Work out the finished part from the listing and answer in its coordinate system (mm). A direction names the side the tool comes from. Round coordinates to 2 decimals unless told otherwise and drop trailing zeros. Order: outer loops, then holes, each group sorted by start corner. A loop starts at its lowest first (then second) coordinate and runs counter-clockwise, first axis right, second up. Notation, with made-up numbers: (82, 39) - (114, 39) arc R20 ccw to (114, 63) - close; hole circle Ø9 at (76, 82). An arc over 180 degrees is marked (long way). Put each result on its own line as item: value.
Solid Edge part; units mm, degrees
sketch "Sketch1" plane through (0, 0, 0) normal (1, 0, 0) x (0, 1, 0)
  circle A0 centre (0, 0) radius 30
  circle A1 centre (0, 0) radius 15
extrude "Protrusion1" add sketch "Sketch1" along normal mid plane 80
sketch "Sketch2" plane through (0, 0, 66) normal (0, 0, 1) x (1, 0, 0)
  line L0 (30, 0) -> (30, 40)
  line L1 (-30, 0) -> (-30, 40)
  line L2 (0, 0) -> (-30, 0)
  line L3 (0, 0) -> (30, 0)
  arc A0 (-30, 40) -> (30, 40) centre (0, 40) cw
extrude "ExtrudedProtrusion_3" add sketch "Sketch2" against normal blind 20
sketch "Sketch3" plane through (0, 0, 0) normal (1, 0, 0) x (0, 1, 0)
  line L0 (0, 46) -> (0, 0)
  line L1 (0, 0) -> (20.4926, 0)
  line L2 (20.4926, 0) -> (20, 22.3607)
  line L3 (20, 46) -> (20, 22.3607)
  line L4 (0, 46) -> (20, 46)
extrude "ExtrudedProtrusion_4" add sketch "Sketch3" along normal mid plane 60
sketch "Sketch4" plane through (0, 0, 0) normal (1, 0, 0) x (0, 1, 0)
  line L0 (0, 66) -> (-26.7217, 13.6364)
  line L1 (-26.7217, 13.6364) -> (-26.7217, 0)
  line L2 (-26.7217, 0) -> (0, 0)
  line L3 (0, 0) -> (0, 66)
extrude "ExtrudedProtrusion_5" add sketch "Sketch4" along normal mid plane 12
sketch "Sketch5" plane through (0, 0, 0) normal (1, 0, 0) x (0, 1, 0)
  circle A0 centre (0, 0) radius 15
extrude "ExtrudedCutout_2" cut sketch "Sketch5" along normal mid plane 321.4657
sketch "Sketch6" plane through (0, 0, 0) normal (1, 0, 0) x (0, 1, 0)
  line L0 (40, 106) -> (60, 106)
  line L1 (60, 106) -> (70, 66)
  line L2 (70, 66) -> (40, 66)
  line L3 (40, 66) -> (40, 106)
revolve "RevolvedProtrusion1" add sketch "Sketch6" angle 360 about axis through (0, 40, 66) along (0, 0, 1)
sketch "Sketch7" plane through (0, 0, 0) normal (1, 0, 0) x (0, 1, 0)
  line L0 (60, 66) -> (50, 106)
  line L1 (50, 106) -> (40, 106)
  line L2 (40, 106) -> (40, 66)
  line L3 (40, 66) -> (60, 66)
revolve "RevolvedCutout1" cut sketch "Sketch7" angle 360 about axis through (0, 40, 106) along (0, 0, -1)
1) A cutting plane is placed at C-C on y = 4. Write down the section's boundary in (x, z).
Findings below:
outline: (-40, -29.73) - (40, -29.73) - (40, -14.46) - (-40, -14.46) - close; (-40, 14.46) - (40, 14.46) - (40, 29.73) - (30, 29.73) - (30, 66) - (-30, 66) - (-30, 29.73) - (-40, 29.73) - close
2) For a pull along Y with two mould halves and no side action, classify faces 5 (the flat face through (0, 7, 66)), 6 (the cylindrical face through (0.56, -14.985, 0.66)), 7 (the cylindrical face through (-0.56, -3.905, -29.745)) as pulls with the +Y half, pulls with the -Y half, needs draft (parallel to the pull), parting line crosses it, or undercut.
Findings below:
face 5: needs draft
face 6: undercut
face 7: parting line crosses it
3) Straight lines are drawn through the part: L1, parallel to Z at x = 16, y = 0.5; L2, parallel to Z at x = -31, y = -9; L3, parallel to Y at x = -10, z = 79.5. For each, find the intervals that lie inside material, in ascending order. Write a range as from..to.
Findings below:
L1: z = -30..-14.99, 14.99..66
L2: z = -28.62..-12, 12..28.62
L3: y = 15.32..26.72, 53.28..64.68
4) A cutting plane is placed at A-A on z = 0. Write down the section's boundary in (x, y).
Findings below:
outline: (-40, -30) - (40, -30) - (40, -15) - (-40, -15) - close; (-40, 15) - (40, 15) - (40, 30) - (-40, 30) - close
5) For faces 1 (the conical face through (4.193, 53.314, 90.164)), 2 (the flat face through (18, 0, 48)), 3 (the flat face through (0, 20, 34)), 4 (the flat face through (-6, -9, 40)), determine the directions among +Z, -Z, +X, -X, +Y, -Y from which every point of the face is accessible in a straight line to the end or side of a thin tool.
Findings below:
face 1: none
face 2: +Z, +X, -Y
face 3: +X, -X, +Y
face 4: +Z, -X, -Y
6) Given pin 1 Ø3 at (x, z) = (-23, 16) entering from -Y; pin 2 Ø7 at (x, z) = (-14, 56) entering from -Y; pin 3 Ø1.5 at (x, z) = (-18.5, -7.5) entering from +Y; pin 4 Ø6 at (y, z) = (21, 23.5) entering from +X, each flat-ended and moving along its own axis, determine where each tip first touches the part or whether it passes through.
Findings below:
pin 1: stops at y = -26.26
pin 2: stops at y = 0
pin 3: stops at y = 29.23
pin 4: stops at x = 40
7) A cutting plane is placed at D-D on z = 80. Write down the section's boundary in (x, y).
Findings below:
outline: circle Ø53 at (0, 40); hole circle Ø33 at (0, 40)
